Verification items for this drawing (mm, ordinates from the low corner). Round coordinates to 2 decimals unless told otherwise and drop trailing zeros. Write each loop counter-clockwise with the first axis right and the second up, starting at its lowest first coordinate (ties: lowest second). Pieces come first, ordered by that corner, then holes.
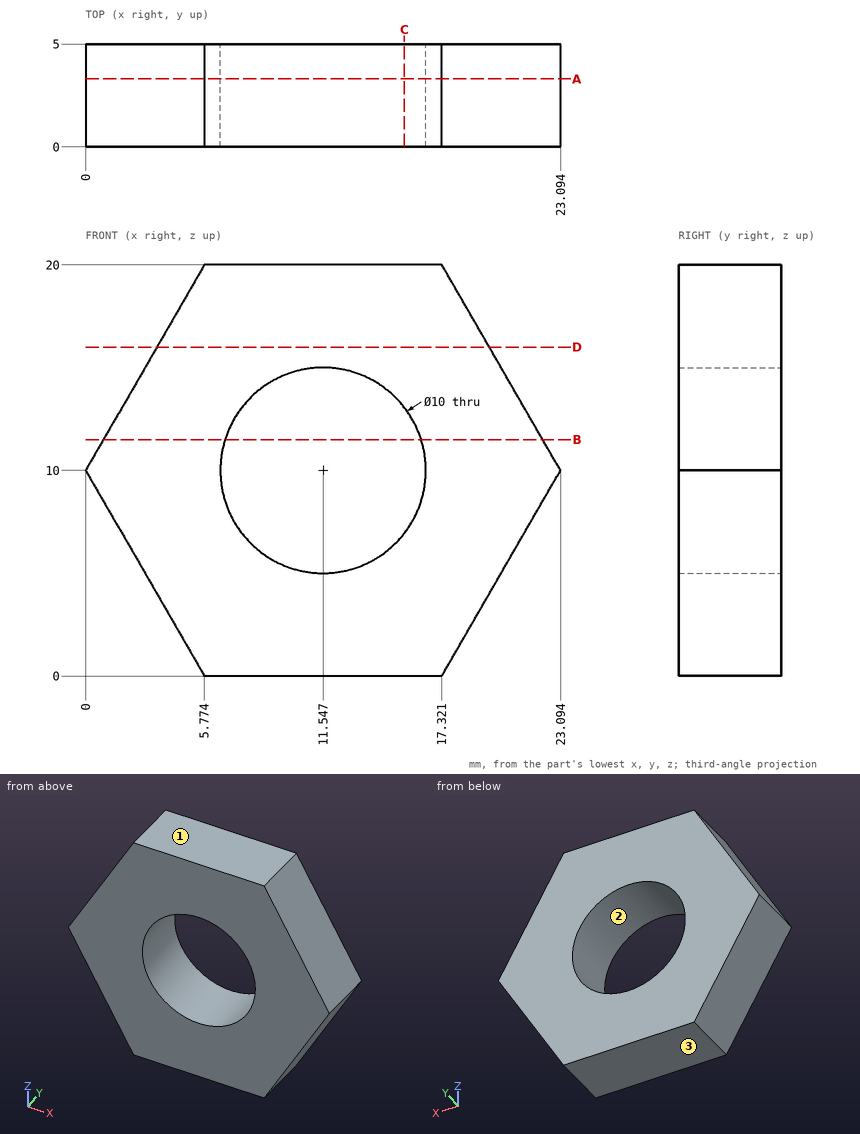
1. Section check D-D (z = 16). Record the cut outline in (x, y) (1 decimal).
2. Depth check by flat-ended pin: pin 1 Ø1.5 at (y, z) = (4, 14) entering from +X; pin 2 Ø1.5 at (y, z) = (3, 15) entering from +X. Enter the tip coordinate at first touch or a pass-through.
3. Section check C-C (x = 15.5). Record the cut outline in (y, z).
4. Section check B-B (z = 11.5). Record the cut outline in (x, y).
5. Release check for a two-part mould opening along Z. For the marked faces 1, 2 and 3 record: +Z half, -Z half, draft (parallel to the pull), parting line (faces both ways), or undercut.
6. Scan lines: line 1 along Z through (x, y) = (15.75, 1.7) (1 decimal); line 2 along Z through (x, y) = (8.25, 3.55); line 3 along X through (y, z) = (3.05, 12) (1 decimal). Record each from-to range of solid material in increasing order.
7. Section check A-A (y = 3.3). Record the cut outline in (x, z) (1 decimal), plus the area to 3 significant figures.
Results below:
1. outline: (3.5, 0) - (19.6, 0) - (19.6, 5) - (3.5, 5) - close
2. pin 1: stops at x = 21.22
2. pin 2: stops at x = 20.64
3. outline: (0, 0) - (5, 0) - (5, 6.94) - (0, 6.94) - close; (0, 13.06) - (5, 13.06) - (5, 20) - (0, 20) - close
4. outline: (0.87, 0) - (6.78, 0) - (6.78, 5) - (0.87, 5) - close; (16.32, 0) - (22.23, 0) - (22.23, 5) - (16.32, 5) - close
5. face 1: +Z half
5. face 2: undercut
5. face 3: -Z half
6. line 1: z = 0 to 7.3, 12.7 to 20
6. line 2: z = 0 to 6.24, 13.76 to 20
6. line 3: x = 1.2 to 7, 16.1 to 21.9
7. outline: (0, 10) - (5.8, 0) - (17.3, 0) - (23.1, 10) - (17.3, 20) - (5.8, 20) - close; hole circle Ø10 at (11.5, 10)
7. area: 268 mm2
